Check sheet for the modelled part. Datum: model origin and axes. Units: mm. Face numbers are marked on the shaded views. Give positions to 0.01 mm unless a question says otherwise; leave off trailing zeros. Order: outer loops, then holes, each group sorted by start corner. A loop starts at its lowest first (then second) coordinate and runs counter-clockwise, first axis right, second up.
```python
from build123d import *

# Parameters (mm, degrees)
SKETCH1_W                    = 72
SKETCH1_H                    = 276
BASE_FLANGE1_DEPTH           = 2
EDGE_FLANGE1_STRIP_W         = 13
EDGE_FLANGE1_STRIP_H         = 2
EDGE_FLANGE1_STRIP_CUT_DEPTH = 276
EDGE_FLANGE1_DEPTH           = 276
EDGE_FLANGE2_STRIP_W         = 13
EDGE_FLANGE2_STRIP_H         = 2
EDGE_FLANGE2_STRIP_CUT_DEPTH = 276
EDGE_FLANGE2_DEPTH           = 276
CUT_EXTRUDE1_DEPTH           = 183.834024801
CUT_EXTRUDE1_DEPTH_BACK      = 183.834024801


# Sheet-metal steps are written as plain solids
with BuildPart() as part:
    # Sketch1 → Base-Flange1 (new body)
    with BuildSketch(Plane.XY):
        with Locations((19.8, 35.625)):
            Rectangle(SKETCH1_W, SKETCH1_H)
    extrude(amount=-BASE_FLANGE1_DEPTH)

    # Edge-Flange1 strip (across the edge) → Edge-Flange1 strip cut (cut)
    with BuildSketch(Plane(origin=(55.8, -102.375, 0), x_dir=(-1, 0, 0), z_dir=(0, 1, 0))):
        with Locations((-2, -1)):
            Rectangle(EDGE_FLANGE1_STRIP_W, EDGE_FLANGE1_STRIP_H)
    extrude(amount=EDGE_FLANGE1_STRIP_CUT_DEPTH, mode=Mode.SUBTRACT)

    # Edge-Flange1 section (across the edge) → Edge-Flange1 (add)
    with BuildSketch(Plane(origin=(55.8, -102.375, 0), x_dir=(-1, 0, 0), z_dir=(0, 1, 0))):
        with BuildLine():
            Line((0, 2.5), (0, 13))
            Line((0, 13), (2, 13))
            Line((2, 13), (2, 2.5))
            ThreePointArc((2, 2.5), (2.732233047, 0.732233047), (4.5, 0))
            Line((4.5, 0), (4.5, -2))
            ThreePointArc((4.5, -2), (1.318019485, -0.681980515), (0, 2.5))
        make_face()
    extrude(amount=EDGE_FLANGE1_DEPTH)

    # Edge-Flange2 strip (across the edge) → Edge-Flange2 strip cut (cut)
    with BuildSketch(Plane(origin=(-16.2, 173.625, 0), x_dir=(1, 0, 0), z_dir=(0, -1, 0))):
        with Locations((-2, -1)):
            Rectangle(EDGE_FLANGE2_STRIP_W, EDGE_FLANGE2_STRIP_H)
    extrude(amount=EDGE_FLANGE2_STRIP_CUT_DEPTH, mode=Mode.SUBTRACT)

    # Edge-Flange2 section (across the edge) → Edge-Flange2 (add)
    with BuildSketch(Plane(origin=(-16.2, 173.625, 0), x_dir=(1, 0, 0), z_dir=(0, -1, 0))):
        with BuildLine():
            Line((0, 2.5), (0, 13))
            Line((0, 13), (2, 13))
            Line((2, 13), (2, 2.5))
            ThreePointArc((2, 2.5), (2.732233047, 0.732233047), (4.5, 0))
            Line((4.5, 0), (4.5, -2))
            ThreePointArc((4.5, -2), (1.318019485, -0.681980515), (0, 2.5))
        make_face()
    extrude(amount=EDGE_FLANGE2_DEPTH)

    # Sketch12 → Cut-Extrude1 (cut, two sides: drawn at the far end of the back side and taken through both)
    with BuildSketch(Plane.XY.offset(-CUT_EXTRUDE1_DEPTH_BACK)):
        with BuildLine():
            Line((26.38258059, 49.625), (26.38258059, 21.625))
            ThreePointArc((26.38258059, 21.625), (20.38258059, 15.625), (14.38258059, 21.625))
            Line((14.38258059, 21.625), (14.38258059, 49.625))
            ThreePointArc((14.38258059, 49.625), (20.38258059, 55.625), (26.38258059, 49.625))
        make_face()
    extrude(amount=CUT_EXTRUDE1_DEPTH + CUT_EXTRUDE1_DEPTH_BACK, mode=Mode.SUBTRACT)


solid = part.part
```
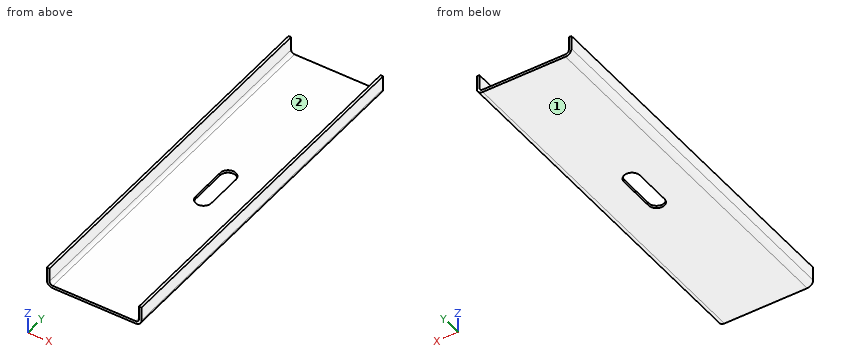
(1) Gauge pin test, flat ends, axial feed: pin 1 Ø8 at (x, y) = (-2.5, 96) entering from +Z; pin 2 Ø1.6 at (y, z) = (36, -1) entering from +X; pin 3 Ø1.6 at (y, z) = (32, -1) entering from -X. Record the tip position at first contact, or that the pin passes through.
Response values:
pin 1: stops at z = 0
pin 2: stops at x = 54.9
pin 3: stops at x = -15.3
(2) Cross-section at B-B on y = 141. Enter the section's corners in (x, z), then the cut area to 3 significant figures.
Response values:
outline: (-16.2, 2.5) arc R4.5 ccw to (-11.7, -2) - (51.3, -2) arc R4.5 ccw to (55.8, 2.5) - (55.8, 13) - (53.8, 13) - (53.8, 2.5) arc R2.5 cw to (51.3, 0) - (-11.7, 0) arc R2.5 cw to (-14.2, 2.5) - (-14.2, 13) - (-16.2, 13) - close
area: 190 mm2
(3) Release check for a two-part mould opening along X. For the marked faces 1 and 2 record: released by +X, released by -X, zero draft, split by the parting line, or undercut.
Response values:
face 1: zero draft
face 2: undercut
(4) Cross-section at C-C on x = 32.5. Enter the section's corners in (y, z) (3 decimals), then the cut area to 3 significant figures.
Response values:
outline: (-102.375, -2) - (173.625, -2) - (173.625, 0) - (-102.375, 0) - close
area: 552 mm2
(5) Material ranges on L1, parallel to X at y = 84, z = 8.75; L2, parallel to Z at x = 31.5, y = 129, recorded low to high.
Response values:
L1: x = -16.2 to -14.2, 53.8 to 55.8
L2: z = -2 to 0
(6) Cross-section at A-A on z = 6.5. Enter the section's corners in (x, y) (3 decimals), then the cut area to 3 significant figures.
Response values:
outline: (-16.2, -102.375) - (-14.2, -102.375) - (-14.2, 173.625) - (-16.2, 173.625) - close; (53.8, -102.375) - (55.8, -102.375) - (55.8, 173.625) - (53.8, 173.625) - close
area: 1,100 mm2
